from build123d import *

# Parameters (mm, degrees)
SKETCH042_R     = 1.5
PAD016_DEPTH    = 20
SKETCH043_R     = 3.1
POCKET016_DEPTH = 3
POCKET017_DEPTH = 7
CHAMFER010_SIZE = 2.4
CHAMFER011_SIZE = 2
PAD018_DEPTH    = 1


with BuildPart() as part:
    # Sketch042 → Pad016 (new body)
    with BuildSketch(Plane.XY):
        Polygon((-5.9, 0), (7.9, 0), (6.9, 6), (6.9, 14), (-1.5, 14), (-1.5, 6), (-3.9, 6), align=None)
        with Locations((1.5, 3)):
            Circle(SKETCH042_R, mode=Mode.SUBTRACT)
    extrude(amount=PAD016_DEPTH)

    # Sketch043 (on Face10 of Pad016) → Pocket016 (cut)
    with BuildSketch(Plane.XY.offset(20)):
        with Locations((1.5, 3)):
            Circle(SKETCH043_R)
    extrude(amount=-POCKET016_DEPTH, mode=Mode.SUBTRACT)

    # Sketch044 (on Face10 of Pocket016) → Pocket017 (cut)
    with BuildSketch(Plane(origin=(0, 14, 0), x_dir=(-1, 0, 0), z_dir=(0, 1, 0))):
        Polygon((-4, 20), (-1.5, 20), (-1.5, 9), (1.5, 9), (1.5, 7), (-4.9, 7), (-4.9, 0), (-6.9, 0), (-6.9, 9), (-4, 9), align=None)
    extrude(amount=-POCKET017_DEPTH, mode=Mode.SUBTRACT)

    # Chamfer010
    chamfer010_edges = [part.edges().sort_by_distance(p)[0] for p in [
        (4, 10.5, 9),
        (1.5, 10.5, 9),
    ]]
    chamfer(chamfer010_edges, length=CHAMFER010_SIZE)

    # Chamfer011
    chamfer011_edges = [part.edges().sort_by_distance(p)[0] for p in [
        (-1.5, 10.5, 7),
    ]]
    chamfer(chamfer011_edges, length=CHAMFER011_SIZE)

    # Sketch046 (on Face17 of Chamfer011) → Pad018 (join)
    with BuildSketch(Plane(origin=(0, 14, 0), x_dir=(-1, 0, 0), z_dir=(0, 1, 0))):
        Polygon((-7, 20), (1.4, 20), (1.4, 0), (-5, 0), (-5, 7), (-7, 9), align=None)
    extrude(amount=-PAD018_DEPTH)


with BuildPart() as part_1:
    # Body008 placement: moved
    add(part.part.moved(Location((0, 21.5, 38))))


solid = part_1.part
Here's how the part is built. I have some questions about the finished solid (model axes, mm). A direction names the side the tool comes from. Coordinates: 2 decimals unless noted, no trailing zeros. Write each loop counter-clockwise with the first axis right and the second up, starting at its lowest first coordinate (ties: lowest second). Pieces come first, ordered by that corner, then holes.
Item 1: I want a section at C-C on y = 31.5. Write out the boundary of the cut face in (x, z), and give its area (3 significant figures).
Item 2: On a 3-axis mill with a long thin cutter (end or side, diameter ignored), from which of +Z, -Z, +X, -X, +Y, -Y can I reach the whole of each face in a straight line? I mean faces 4 (the flat face through (5, 35, 41)), 5 (the flat face through (-0.5, 31.3, 44)), 6 (the flat face through (5.2, 31.5, 48.2)), 7 (the flat face through (7, 35, 52)). Say none if no direction works.
Item 3: I want a section at A-A on y = 24.5. Write out the boundary of the cut face in (x, z), and give its area (3 significant figures).
Item 4: If we mould it in two halves opening along X, with no side actions, what happens to faces 1 (the flat face through (-1.5, 32, 48)), 2 (the flat face through (4, 32, 54)), 3 (the flat face through (1, 29, 58))? For each: +X half, -X half, draft (parallel to the pull), parting line (faces both ways), or undercut.
Item 5: Will these pins go through, and if not, where does the flat tip stop? pin 1 (6.5 mm diameter, centred on y = 32, z = 52, fed in from -X); pin 2 (5.5 mm diameter, centred on x = 1.5, y = 24.5, fed in from +Z); pin 3 (1.5 mm diameter, centred on y = 34, z = 53.5, fed in from +X).
Item 6: I want a section at B-B on z = 42.25. Write out the boundary of the cut face in (x, y), and give its area (3 significant figures).
Item 7: I want a section at D-D on z = 51. Write out the boundary of the cut face in (x, y), and give its area (3 significant figures).
Item 8: If I drill on line 1 (Y direction, x = 1.5, z = 46.25); line 2 (X direction, y = 30, z = 52.5); line 3 (Y direction, x = 1.5, z = 44), over which ranges is the centre line in solid material (lowest first)?
Findings below:
1. outline: (-1.5, 38) - (4.9, 38) - (4.9, 45) - (0.5, 45) - (-1.5, 43) - close; (-1.5, 47) - (-0.9, 47) - (1.5, 49.4) - (1.5, 58) - (-1.5, 58) - close; (4, 49.4) - (6.4, 47) - (6.9, 47) - (6.9, 58) - (4, 58) - close
1. area: 102 mm2
2. face 4: -Z, +X, +Y
2. face 5: -X
2. face 6: none
2. face 7: +Z, -Z, +X, +Y
3. outline: (-4.9, 38) - (0, 38) - (0, 55) - (-1.6, 55) - (-1.6, 58) - (-4.9, 58) - close; (3, 38) - (7.4, 38) - (7.4, 58) - (4.6, 58) - (4.6, 55) - (3, 55) - close
3. area: 176 mm2
4. face 1: -X half
4. face 2: undercut
4. face 3: draft
5. pin 1: stops at x = -1.5
5. pin 2: stops at z = 55
5. pin 3: stops at x = 7
6. outline: (-5.9, 21.5) - (7.9, 21.5) - (6.9, 27.5) - (6.9, 28.5) - (4.9, 28.5) - (4.9, 34.5) - (5, 34.5) - (5, 35.5) - (-1.5, 35.5) - (-1.5, 27.5) - (-3.9, 27.5) - close; hole circle Ø3 at (1.5, 24.5)
6. area: 120 mm2
7. outline: (-5.9, 21.5) - (7.9, 21.5) - (6.9, 27.5) - (6.9, 34.5) - (7, 34.5) - (7, 35.5) - (-1.5, 35.5) - (-1.5, 27.5) - (-3.9, 27.5) - close; hole circle Ø3 at (1.5, 24.5); hole (1.5, 28.5) - (4, 28.5) - (4, 34.5) - (1.5, 34.5) - close
7. area: 119 mm2
8. line 1: y = 21.5 to 23, 26 to 28.5, 34.5 to 35.5
8. line 2: x = -1.5 to 1.5, 4 to 6.9
8. line 3: y = 21.5 to 23, 26 to 35.5
